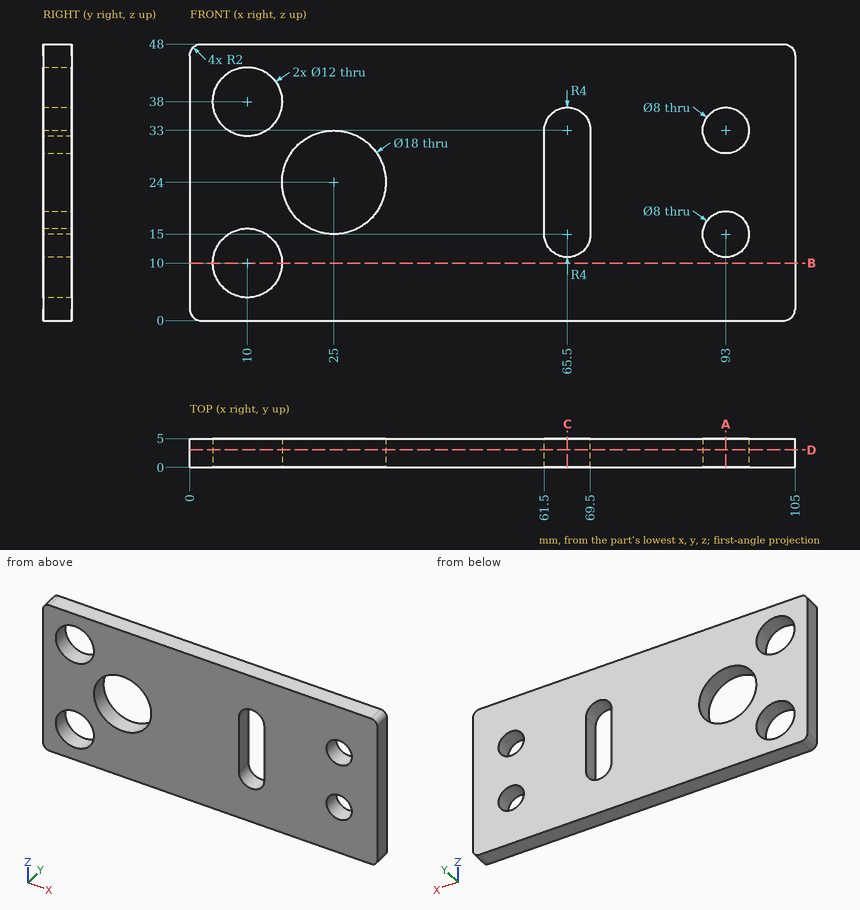
Geometry: see drawing. Coordinates: mm, zero at the bounding-box minimum. Round coordinates to 2 decimals unless told otherwise and drop trailing zeros. Loops run counter-clockwise (first coordinate to the right, second up) from the corner with the lowest first, then second, coordinate; pieces in that order, holes last.
(1) Section query A-A (x = 93). Output: boundary loops of the cut face in (y, z), and give its area (3 significant figures).
From the geometry:
outline: (0, 0) - (5, 0) - (5, 11) - (0, 11) - close; (0, 19) - (5, 19) - (5, 29) - (0, 29) - close; (0, 37) - (5, 37) - (5, 48) - (0, 48) - close
area: 160 mm2
(2) Material intervals for probe 1 along X at (y, z) = (3.95, 24); probe 2 along X at (y, z) = (2.75, 10); probe 3 along Z at (x, y) = (9, 0.85), sorted ascending.
From the geometry:
probe 1: x = 0 to 16, 34 to 61.5, 69.5 to 105
probe 2: x = 0 to 4, 16 to 105
probe 3: z = 0 to 4.08, 15.92 to 32.08, 43.92 to 48
(3) Section query D-D (y = 3.05). Output: boundary loops of the cut face in (x, z).
From the geometry:
outline: (0, 2) arc R2 ccw to (2, 0) - (103, 0) arc R2 ccw to (105, 2) - (105, 46) arc R2 ccw to (103, 48) - (2, 48) arc R2 ccw to (0, 46) - close; hole circle Ø12 at (10, 10); hole circle Ø12 at (10, 38); hole circle Ø18 at (25, 24); hole (61.5, 15) arc R4 ccw to (69.5, 15) - (69.5, 33) arc R4 ccw to (61.5, 33) - close; hole circle Ø8 at (93, 15); hole circle Ø8 at (93, 33)
(4) Section query C-C (x = 65.5). Output: boundary loops of the cut face in (y, z), and give its area (3 significant figures).
From the geometry:
outline: (0, 0) - (5, 0) - (5, 11) - (0, 11) - close; (0, 37) - (5, 37) - (5, 48) - (0, 48) - close
area: 110 mm2
(5) Contact query for a flat-ended pin moving along its axis: pin 1 Ø8 at (x, z) = (28.5, 23) entering from +Y. Output: stop coordinate, or through.
From the geometry:
pin 1: passes through
(6) Section query B-B (z = 10). Output: boundary loops of the cut face in (x, y), and give its area (3 significant figures).
From the geometry:
outline: (0, 0) - (4, 0) - (4, 5) - (0, 5) - close; (16, 0) - (105, 0) - (105, 5) - (16, 5) - close
area: 465 mm2
